from build123d import *

# Parameters (mm, degrees)
F0_W     = 200
F0_H     = 200
F1_DEPTH = 15
F2_R     = 2.165
F3_DEPTH = 50
F4_R     = 2.165
F5_DEPTH = 50


with BuildPart() as f1:
    # F0 (on Top) → F1 (new body)
    with BuildSketch(Plane.XY):
        Rectangle(F0_W, F0_H)
    extrude(amount=F1_DEPTH)

    # F2 (on face) → F3 (join)
    with BuildSketch(Plane(origin=(0, 100, 0), x_dir=(-1, 0, 0), z_dir=(0, 1, 0))):
        with Locations((-91.25, 7.5)):
            Circle(F2_R)
        with Locations((91.25, 7.5)):
            Circle(F2_R)
    extrude(amount=F3_DEPTH)

    # F4 (on face) → F5 (join)
    with BuildSketch(Plane.XZ.offset(100)):
        with Locations((-91.25, 7.5)):
            Circle(F4_R)
        with Locations((91.25, 7.5)):
            Circle(F4_R)
    extrude(amount=F5_DEPTH)


solid = f1.part
Model file for the job. Use its own axes, mm. Give positions to 0.01 mm unless a question says otherwise; leave off trailing zeros. Order: outer loops, then holes, each group sorted by start corner. A loop starts at its lowest first (then second) coordinate and runs counter-clockwise, first axis right, second up. Notation, with made-up numbers: (83, 66) - (141, 66) arc R18 ccw to (141, 74) - close; hole circle Ø2 at (59, 31). An arc over 180 degrees is marked (long way). One line per item, written item: value.
Item 1: Slice it at A-A (y = 112.5). List the corners of the cut face in (x, z) (3 decimals), then the cut area to 3 significant figures.
Response values:
outline: circle Ø4.33 at (-91.25, 7.5); circle Ø4.33 at (91.25, 7.5)
area: 29.5 mm2
Item 2: Pin check, flat tips, straight feed: pin 1 Ø1.5 at (x, z) = (19, 2) entering from +Y; pin 2 Ø5 at (x, z) = (5, 4.5) entering from -Y; pin 3 Ø1.5 at (y, z) = (-105, 8.5) entering from +X. Stop position of each tip, or through.
Response values:
pin 1: y = 100
pin 2: y = -100
pin 3: x = 93.4
Item 3: Two-plate mould, pull along X, no slides. Class faces 1 (the flat face through (100, -1, 7)), 2 (the flat face through (-1, 100, 7)), 3 (the flat face through (-1, 1, 15)): released by +X, released by -X, zero draft, split by the parting line, or undercut.
Response values:
face 1: released by +X
face 2: undercut
face 3: zero draft
Item 4: Wall check: line 1 (Y direction, x = -83, z = 13). Give the ranges that are in metal, low to high.
Response values:
line 1: -100 to 100
Item 5: Slice it at B-B (x = 76.5). List the corners of the cut face in (y, z), then the cut area to 3 significant figures.
Response values:
outline: (-100, 0) - (100, 0) - (100, 15) - (-100, 15) - close
area: 3,000 mm2
